```python
from build123d import *

# Parameters (mm, degrees)
BOSS_EXTRUDE1_DEPTH = 30
SKETCH2_R           = 12.5
CUT_EXTRUDE1_DEPTH  = 60
SKETCH4_R           = 12.5
BOSS_EXTRUDE2_DEPTH = 10


with BuildPart() as part:
    # Sketch1 → Boss-Extrude1 (new body, symmetric)
    with BuildSketch(Plane(origin=(0, 0, 0), x_dir=(1, 0, 0), z_dir=(0, 1, 0))):
        Polygon((0, -6.5), (73.516660498, -6.5), (139.782032303, -44.758330249), (146.282032303, -33.5), (77, 6.5), (0, 6.5), align=None)
    extrude(amount=BOSS_EXTRUDE1_DEPTH, both=True)

    # Sketch2 → Cut-Extrude1 (cut)
    with BuildSketch(Plane(origin=(22.064582562, 0, -38.216978046), x_dir=(-0.866025404, 0, -0.5), z_dir=(0.5, 0, -0.866025404))):
        with Locations((-113.433956091, 0)):
            Circle(SKETCH2_R)
        with BuildLine():
            Line((-143.433956091, 30), (-143.433956091, 2.09e-07))
            ThreePointArc((-143.433956091, 2.09e-07), (-134.647159453, 21.21320351), (-113.433956091, 30))
            Line((-113.433956091, 30), (-143.433956091, 30))
        make_face()
        with BuildLine():
            Line((-143.433956091, 2.09e-07), (-143.433956091, -30))
            Line((-143.433956091, -30), (-113.433956091, -30))
            ThreePointArc((-113.433956091, -30), (-134.647159601, -21.213203362), (-143.433956091, 2.09e-07))
        make_face()
    extrude(amount=-CUT_EXTRUDE1_DEPTH, mode=Mode.SUBTRACT)

    # Sketch4 → Boss-Extrude2 (add)
    with BuildSketch(Plane(origin=(31.02146997, 17.910254038, -9.598076211), x_dir=(0.5, -0.866025404, 0), z_dir=(0.836516304, 0.482962913, -0.258819045))):
        with BuildLine():
            Line((-13.480762114, -3.207364507), (41.519237886, -3.207364507))
            Line((41.519237886, -3.207364507), (41.519237886, 28.792635493))
            ThreePointArc((41.519237886, 28.792635493), (14.019237886, 56.292635493), (-13.480762114, 28.792635493))
            Line((-13.480762114, 28.792635493), (-13.480762114, -3.207364507))
        make_face()
        with Locations((14.019237886, 28.792635493)):
            Circle(SKETCH4_R, mode=Mode.SUBTRACT)
    extrude(amount=-BOSS_EXTRUDE2_DEPTH)


solid = part.part
```
Here's how the part is built. I have some questions about the finished solid (model axes, mm). A direction names the side the tool comes from. Coordinates: 2 decimals unless noted, no trailing zeros. Write each loop counter-clockwise with the first axis right and the second up, starting at its lowest first coordinate (ties: lowest second). Pieces come first, ordered by that corner, then holes. Notation, with made-up numbers: (60, -2) - (98, -2) arc R31 ccw to (98, 34) - close; hole circle Ø4 at (-32, -21.5). An arc over 180 degrees is marked (long way). One line per item, written item: value.
1) I need wall thicknesses on line 1 along X through (y, z) = (24, 8.5); line 2 along Z through (x, y) = (13, 23.5); line 3 along Z through (x, y) = (18, 1). Which ranges of each line are inside material? Lowest first, please.
Model answer:
line 1: x = 76.98 to 102.98
line 2: z = -6.5 to 6.5
line 3: z = -61.93 to -45.54, -6.5 to 6.5
2) Suppose I cut it at B-B on y = -5. State how many separate pieces and enclosed holes the cut face has, and give its area (3 significant figures).
Model answer:
separate pieces: 3
enclosed holes: 0
area: 2,110 mm²
3) We'd pull the mould along Y, two halves only. Please class faces 1 (the flat face through (44.84, -22.054, -20.462)), 2 (the cylindrical face through (106.77, 3.75, 18.09)), 3 (the cylindrical face through (21.59, -4.42, -62.69)), 4 (the cylindrical face through (24.2, 9.24, -28.79)): pulls with the +Y half, pulls with the -Y half, needs draft (parallel to the pull), parting line crosses it, or undercut.
Model answer:
face 1: pulls with the -Y half
face 2: undercut
face 3: parting line crosses it
face 4: undercut
4) Suppose I cut it at A-A on x = 50. Write out the boundary of the cut face in (y, z).
Model answer:
outline: (-30, -6.5) - (-19.07, -6.5) - (-19.07, -17.27) - (-13.3, -6.5) - (30, -6.5) - (30, 6.5) - (-30, 6.5) - close
5) I'm going to push flat-ended pins straight in: P1, Ø10, axis at x = 16, y = -11.5, coming from the +Z side; P2, Ø2, axis at x = 44.5, z = -31, coming from the +Y side; P3, Ø10, axis at x = 106, y = -2, coming from the -Z side. Where does each tip first touch, or does it pass through?
Model answer:
P1: stops at z = 6.5
P2: stops at y = -15.09
P3: stops at z = 7.36
6) Suppose I cut it at C-C on x = 70. Write out the boundary of the cut face in (y, z), and give its area (3 significant figures).
Model answer:
outline: (-30, -6.5) - (30, -6.5) - (30, 6.5) - (-30, 6.5) - close
area: 780 mm²
7) On a 3-axis mill with a long thin cutter (end or side, diameter ignored), from which of +Z, -Z, +X, -X, +Y, -Y can I reach the whole of each face in a straight line? I mean faces 5 (the flat face through (17.24, 25.52, -20.9)), 6 (the flat face through (26, -0.8, -22.1)), 7 (the flat face through (36, 0, 6.5)), 8 (the flat face through (39, 7, -6.5)). Say none if no direction works.
Model answer:
face 5: -Z, -X, +Y
face 6: -X, -Y
face 7: +Z, -X, +Y, -Y
face 8: none
